Work out the finished part from the listing and answer in its coordinate system (mm). A direction names the side the tool comes from. Coordinates: 2 decimals unless noted, no trailing zeros. Order: outer loops, then holes, each group sorted by start corner. A loop starts at its lowest first (then second) coordinate and runs counter-clockwise, first axis right, second up. Notation, with made-up numbers: M -37.5,-31 L -29.5,-31 A29 cw -29.5,-5 Z; hole C 49.5,-27.75 d8. An arc over 180 degrees is marked long. Write item = value, one per line. Start each with the question number.
Q1. Find section D-D on x = -3. Give the vertices of the cut face in (y, z).
Q2. Straight lines are drawn through the part: line 1 along Z through (x, y) = (-4.25, 4); line 2 along X through (y, z) = (0, -2.5); line 3 along X through (y, z) = (-1.75, -2.5). For each, find the intervals that lie inside material, in ascending order.
Q3. Each of these flat-tipped pins is pushed along its axis until it touches: P1, Ø3, axis at x = -2, y = 0.5, coming from the -Z side; P2, Ø3, axis at y = -2.5, z = -3, coming from the -X side; P3, Ø3, axis at x = -4.5, y = -3, coming from the -Z side. Where does it stop, or does it pass through?
Q4. Find section B-B on z = -1.5. Give the vertices of the cut face in (x, y).
Q5. Determine the mould class of faces 6 (the cylindrical face through (-5.263, -0.243, 1.014)), 7 (the cylindrical face through (1.617, -0.67, 0.493)), 8 (the flat face through (-2.4, 2.4, 2)) for opening direction Y: released by +Y, released by -Y, zero draft, split by the parting line, or undercut.
Q6. A tool of negligible diameter and unlimited length cuts with its end or side. For faces 1 (the cylindrical face through (1.25, 4.41, -4.81)), 2 (the cylindrical face through (-6.699, 0.285, 1.014)), 3 (the cylindrical face through (2.92, -2.76, -2.46)), 4 (the cylindrical face through (-4.1, -1.01, -2.5)), 5 (the cylindrical face through (1.01, 4.1, -2.5)), from which of +Z, -Z, +X, -X, +Y, -Y can it reach the whole face along a straight path? Write none if from no direction.
Q7. Find section A-A on z = 0.25. Give the vertices of the cut face in (x, y), and give its area (3 significant figures).
```python
from build123d import *

# Parameters (mm, degrees)
SKETCH_R     = 1.75
PAD_DEPTH    = 2
FILLET_R     = 1
CHAMFER_SIZE = 1
PAD001_DEPTH = 5
FILLET001_R  = 1


with BuildPart() as part:
    # Sketch → Pad (new body)
    with BuildSketch(Plane.XY):
        with BuildLine():
            ThreePointArc((-5, 0), (3.535534, -3.535534), (0, 5))
            Line((0, 7), (0, 5))
            Line((-7, 7), (0, 7))
            Line((-7, 0), (-7, 7))
            Line((-5, 0), (-7, 0))
        make_face()
        Circle(SKETCH_R, mode=Mode.SUBTRACT)
    extrude(amount=PAD_DEPTH)

    # Fillet
    fillet_edges = [part.edges().sort_by_distance(p)[0] for p in [
        (-7, 0, 1),
        (-7, 7, 1),
        (0, 7, 1),
        (0, 5, 1),
        (-5, 0, 1),
    ]]
    fillet(fillet_edges, radius=FILLET_R)

    # Chamfer
    chamfer_edges = [part.edges().sort_by_distance(p)[0] for p in [
        (-1.75, 0, 2),
    ]]
    chamfer(chamfer_edges, length=CHAMFER_SIZE)

    # Sketch001 (on Face14 of Chamfer) → Pad001 (join)
    with BuildSketch(Plane(origin=(0, 0, 0), x_dir=(1, 0, 0), z_dir=(0, 0, -1))):
        with BuildLine():
            ThreePointArc((0.833333, -3.930066), (2.840763, 2.840763), (-3.930066, 0.833333))
            Line((-4.930066, 0.833333), (-3.930066, 0.833333))
            ThreePointArc((0.833333, -4.930066), (3.535534, 3.535534), (-4.930066, 0.833333))
            Line((0.833333, -3.930066), (0.833333, -4.930066))
        make_face()
    extrude(amount=PAD001_DEPTH)

    # Fillet001
    fillet001_edges = [part.edges().sort_by_distance(p)[0] for p in [
        (-4.430066, -0.833333, -5),
        (0.833333, 4.430066, -5),
        (0.833333, 3.930066, -2.5),
        (-3.930066, -0.833333, -2.5),
    ]]
    fillet(fillet001_edges, radius=FILLET001_R)


solid = part.part
```
Findings below:
q1.outline = M -4,-5 L -2.67,-5 L -2.67,0 L 7,0 L 7,2 L -4,2 Z
q2.line_1 = 0 to 2
q2.line_2 = 4.02 to 5
q2.line_3 = -4.68 to -3.62, 3.62 to 4.68
q3.P1 = 0
q3.P2 = -4.9
q3.P3 = -5
q4.outline = M -4.93,-0.83 A5 ccw long 0.83,4.93 L 0.83,4.67 A1 ccw 1.47,3.74 A4.02 cw long -3.74,-1.47 A1 ccw -4.67,-0.83 Z
q5.face_6 = released by -Y
q5.face_7 = undercut
q5.face_8 = zero draft
q6.face_1 = -Z, -X, +Y
q6.face_2 = +Z, -Z, -X, -Y
q6.face_3 = -Z
q6.face_4 = -Z, +Y
q6.face_5 = -Z, -X
q7.outline = M -7,1 A1 ccw -6,0 L -5.92,0 A1 cw -4.93,-0.83 A5 ccw long 0.83,4.93 A1 cw 0,5.92 L 0,6 A1 ccw -1,7 L -6,7 A1 ccw -7,6 Z; hole C 0,0 d3.5
q7.area = 98.0 mm^2
